Part model, mm, in its own coordinate system. A direction names the side the tool comes from. Coordinates: 2 decimals unless noted, no trailing zeros. Loops run counter-clockwise (first coordinate to the right, second up) from the corner with the lowest first, then second, coordinate; pieces in that order, holes last. Notation, with made-up numbers: (35, 57) - (56, 57) arc R17 ccw to (56, 64) - close; hole circle Ø2 at (34.25, 11.25). An arc over 180 degrees is marked (long way). Use a Markdown table: item, result. Add a question column.
1. 3-axis set-ups, long thin cutter, end or side, ignore diameter. For faces 1 (the flat face through (-2, 0, 4)), 2 (the cylindrical face through (5.84, -0.54, -2.44)): which of +Z, -Z, +X, -X, +Y, -Y reach the whole face in a straight line?
2. Drop a flat-ended pin along its axis: pin 1 (2 mm diameter, centred on x = 5.5, y = -2.5, fed in from -Z). Give the stop position or say it passes through.
3. Band-saw the part on C-C, the plane x = -0.25. Give the cut face in (y, z), plus the area to 3 significant figures.
4. Wall check: probe 1 along X at (y, z) = (-2.5, 2.25); probe 2 along Z at (x, y) = (7.5, 0); probe 3 along Z at (x, y) = (6.75, -0.75). Give the ranges that are in metal, low to high. Write a range as [from, to].
5. Band-saw the part on A-A, the plane x = -2. Give the cut face in (y, z).
6. Band-saw the part on B-B, the plane x = 11. Give the cut face in (y, z), plus the area to 3 significant figures.
Autodesk Inventor part; units mm, degrees
ref_plane "Work Plane1" through (1.525, 0, 0) normal (0, 0, 1) x (1, 0, 0)
ref_plane "YZ Plane" through (0, 0, 0) normal (1, 0, 0) x (0, 1, 0)
ref_plane "XZ Plane" through (0, 0, 0) normal (0, 1, 0) x (-1, 0, 0)
sketch "Sketch1" plane through (0, 0, 0) normal (0, 0, 1) x (1, 0, 0)
  line L0 (0, 3.44) -> (0, 2.5)
  line L1 (2.4, 2.5) -> (12, 2.5)
  line L2 (12, 2.5) -> (12, 0)
  line L3 (12, 0) -> (-0.5001, 0)
  line L4 (-3.0001, 0) -> (14.5, 0)
  line L5 (-0.5001, 0) -> (-0.5001, 3.44)
  line L6 (-0.5001, 3.44) -> (0, 3.44)
  line L7 (2.4, 2.5) -> (1.9091, 2.5)
  line L8 (1.9091, 2.5) -> (0, 2.5)
  line L9 (0, -0.688) -> (0, 4.128)
  dimension "d0" = 12
  dimension "d1" = 9.6
  dimension "d2" = 5
  dimension "d9" = 0.5001
  dimension "d10" = 6.88
  dimension "d13" = 0.4909
  dimension "d14" = 5
revolve "Body" add sketch "Sketch1" angle 360 about axis through (12, 0, 0) along (-1, 0, 0)
sketch "Sketch2" plane through (-0.5001, 0, 0) normal (-1, 0, 0) x (0, 0, 1)
  line L0 (0, 4.6188) -> (4, 2.3094)
  line L1 (4, 2.3094) -> (4, -2.3094)
  line L2 (4, -2.3094) -> (0, -4.6188)
  line L3 (0, -4.6188) -> (-4, -2.3094)
  line L4 (-4, -2.3094) -> (-4, 2.3094)
  line L5 (-4, 2.3094) -> (0, 4.6188)
  point P0 (0, 0)
  point P1 (0, 0)
  dimension "d11" = 8
extrude "Head" add sketch "Sketch2" along normal blind 3
sketch "Sketch4" plane through (0, 0, 0) normal (0, 0, 1) x (1, 0, 0)
  line L0 (-3.5001, 4) -> (-3.5001, 4.6188)
  line L1 (-3.5001, 4.6188) -> (-3.1428, 4.6188)
  line L2 (-3.1428, 4.6188) -> (-3.5001, 4)
  line L3 (-4.1001, 0) -> (0.0999, 0)
  line L4 (-0.5001, 4.6188) -> (-3.5001, 4.6188)
  line L5 (-3.5001, 2.3094) -> (-3.5001, 4.6188)
  dimension "d5" = 30
  dimension "d19" = 8
revolve "Chamfer1" cut sketch "Sketch4" angle 360 about axis through (-10, 0, 0) along (1, 0, 0)
thread "Thread"
chamfer "Chamfer2" distance 0.4908 distance2 0.4909 1 edges at (12, -2.5, 0) measured on face at (12, -0.7379, 0.3873)
ref_plane "Work Plane1" through (1.525, 0, 0) normal (0, 0, 1) x (1, 0, 0)
equation "\"d0\" = NLG"
equation "\"d1\" = GEL"
equation "\"d2\" = GD"
equation "\"d10\" = SD2"
equation "\"d14\" = BDM"
equation "\"d11\" = SW"
equation "\"d3\" = KOH - SD"
equation "\"d5\" = ANG1"
equation "\"d19\" = SW0"
equation "\"d15\" = GEL"
equation "\"d6\" = -0.5 * SPD + 0.5 * GD"
equation "\"NLG\" = 12"
equation "\"GD\" = NND"
equation "\"BDM\" = NND"
equation "\"KOH\" = 3.5"
equation "\"GEL\" = 9.6"
equation "\"SW\" = 8"
equation "\"SW0\" = SW"
equation "\"SPD\" = NND - 1.2269 * PTC"
equation "\"SD2\" = 6.88"
equation "\"SD\" = 0.5"
equation "\"ANG1\" = 30deg"
equation "\"GAL\" = 0.61345 * PTC"
equation "\"GUL\" = 0.61345 * PTC"
equation "\"RR\" = 0.2"
equation "\"GD1\" = THREADDIA - 1.2269 * PTC"
equation "\"THREADDIA\" = 5"
equation "\"SDH\" = SD2"
equation "\"SDHG\" = 2.4"
equation "\"TOA\" = 30deg"
equation "\"PTC\" = 0.8"
equation "\"NND\" = 5"
equation "\"E0\" = 9.24"
properties part number "ISO 4017 - M5 x 12" material "Steel, Mild"
Geometry check:
| question | item | result |
|---|---|---|
| 1 | face 1 | +Z, +X, -X, +Y, -Y |
| 1 | face 2 | +X |
| 2 | pin 1 | stops at z = -2 |
| 3 | outline | circle Ø6.88 at (0, 0) |
| 3 | area | 37.2 mm^2 |
| 4 | probe 1 | x = [-3.5, 0] |
| 4 | probe 2 | z = [-2.5, 2.5] |
| 4 | probe 3 | z = [-2.38, 2.38] |
| 5 | outline | (-4.62, 0) - (-2.31, -4) - (2.31, -4) - (4.62, 0) - (2.31, 4) - (-2.31, 4) - close |
| 6 | outline | circle Ø5 at (0, 0) |
| 6 | area | 19.6 mm^2 |
